from build123d import *

# Parameters (mm, degrees)
F0_W     = 12.7
F0_H     = 127
F1_DEPTH = 63.5
F2_R     = 9.525
F2_R_2   = 3.175
F3_DEPTH = 12.701


with BuildPart() as f1:
    # F0 (on Front) → F1 (new body, symmetric)
    with BuildSketch(Plane.XZ):
        Rectangle(F0_W, F0_H)
    extrude(amount=F1_DEPTH, both=True)

    # F2 (on face) → F3 (cut, through all)
    with BuildSketch(Plane(origin=(-6.35, 0, 0), x_dir=(0, -1, 0), z_dir=(-1, 0, 0))):
        with Locations((0, 12.7)):
            Circle(F2_R)
        with Locations((-12.7, 25.4)):
            Circle(F2_R_2)
        with Locations((-12.7, 0)):
            Circle(F2_R_2)
        with Locations((12.7, 0)):
            Circle(F2_R_2)
        with Locations((12.7, 25.4)):
            Circle(F2_R_2)
        with Locations((-31.75, -37.1475)):
            Circle(F2_R_2)
        with Locations((31.75, -37.1475)):
            Circle(F2_R_2)
    extrude(amount=-F3_DEPTH, mode=Mode.SUBTRACT)


solid = f1.part
Source: CAD feature listing. Evaluate the final solid. Frame: model axes, mm. Round coordinates to 2 decimals unless told otherwise and drop trailing zeros. Loops run counter-clockwise (first coordinate to the right, second up) from the corner with the lowest first, then second, coordinate; pieces in that order, holes last. Notation, with made-up numbers: (10.25, 38.25) - (28.25, 38.25) arc R14 ccw to (28.25, 52.25) - close; hole circle Ø3 at (48, 25.5). An arc over 180 degrees is marked (long way). Write item = value, one per line. Start each with the question number.
Item 1: Mould query, pull axis Y, two halves, no side actions, for faces 1 (the face through (0, -1, -63.5)), 2 (the face through (-0.09, 9.67, 0.95)), 3 (the face through (0, 63.5, 1)). Classes: released by +Y, released by -Y, zero draft, split by the parting line, or undercut.
Item 2: Section query C-C on y = 12.7. Output: boundary loops of the cut face in (x, z) (3 decimals).
Item 3: Section query B-B on z = 12.7. Output: boundary loops of the cut face in (x, y) (3 decimals), plus the area to 3 significant figures.
Item 4: Material intervals for line 1 (Z direction, x = -0.5, y = -12.7) (3 decimals); line 2 (Z direction, x = -2.25, y = 0) (3 decimals); line 3 (Y direction, x = -1, z = -36.5), sorted ascending.
Item 5: First-contact query: pin 1 Ø7.5 at (y, z) = (-12.7, 25.4) entering from +X. Flat tip, straight axial feed; report the tip coordinate or a pass-through.
Item 6: Section query A-A on y = 31.75. Output: boundary loops of the cut face in (x, z).
Item 7: Section query D-D on x = -2.75. Count the separate pieces of the cut face and the enclosed holes in it, plus the area to 3 significant figures.
Results list:
q1.face_1 = zero draft
q1.face_2 = undercut
q1.face_3 = released by +Y
q2.outline = (-6.35, -63.5) - (6.35, -63.5) - (6.35, -3.175) - (-6.35, -3.175) - close; (-6.35, 3.175) - (6.35, 3.175) - (6.35, 22.225) - (-6.35, 22.225) - close; (-6.35, 28.575) - (6.35, 28.575) - (6.35, 63.5) - (-6.35, 63.5) - close
q3.outline = (-6.35, -63.5) - (6.35, -63.5) - (6.35, -9.525) - (-6.35, -9.525) - close; (-6.35, 9.525) - (6.35, 9.525) - (6.35, 63.5) - (-6.35, 63.5) - close
q3.area = 1,370 mm²
q4.line_1 = -63.5 to -3.175, 3.175 to 22.225, 28.575 to 63.5
q4.line_2 = -63.5 to 3.175, 22.225 to 63.5
q4.line_3 = -63.5 to -34.86, -28.64 to 28.64, 34.86 to 63.5
q5.pin_1 = 6.35
q6.outline = (-6.35, -63.5) - (6.35, -63.5) - (6.35, -40.32) - (-6.35, -40.32) - close; (-6.35, -33.97) - (6.35, -33.97) - (6.35, 63.5) - (-6.35, 63.5) - close
q7.separate_pieces = 1
q7.enclosed_holes = 7
q7.area = 15,700 mm²
